```python
from build123d import *

# Parameters (mm, degrees)
F3_DEPTH = 10
F4_R     = 15
F5_DEPTH = 52.4
F6_W     = 100
F6_H     = 6
F7_DEPTH = 18
F8_R     = 10


with BuildPart() as f1:
    # F0 (on Top) → F1 (revolve)
    with BuildSketch(Plane.XY):
        Polygon((-50, 0), (0, 0), (0, 50), (-20, 50), (-20, 30), (-50, 30), align=None)
    revolve(axis=Axis((-25, 0, 0), (1, 0, 0)))

    # F2 (on face) → F3 (cut)
    with BuildSketch(Plane.YZ):
        with BuildLine():
            Line((49.638695, 6), (-49.638695, 6))
            ThreePointArc((-49.638695, 6), (-49.909592, 3.005434), (-50, 0))
            ThreePointArc((-50, 0), (-49.909592, -3.005434), (-49.638695, -6))
            Line((-49.638695, -6), (49.638695, -6))
            ThreePointArc((49.638695, -6), (49.909592, -3.005434), (50, 0))
            ThreePointArc((50, 0), (49.909592, 3.005434), (49.638695, 6))
        make_face()
    extrude(amount=-F3_DEPTH, mode=Mode.SUBTRACT)

    # F4 (on face) → F5 (cut)
    with BuildSketch(Plane(origin=(-50, 0, 0), x_dir=(0, -1, 0), z_dir=(-1, 0, 0))):
        Circle(F4_R)
    extrude(amount=-F5_DEPTH, mode=Mode.SUBTRACT)

    # F6 (on Front) → F7 (cut)
    with BuildSketch(Plane.XZ):
        Rectangle(F6_W, F6_H)
    extrude(amount=-F7_DEPTH, mode=Mode.SUBTRACT)

    # F8
    f8_edges = [f1.edges().sort_by_distance(p)[0] for p in [
        (-20, -30, 0),
    ]]
    fillet(f8_edges, radius=F8_R)


solid = f1.part
```
The listing builds one solid part. Answer for the finished solid, in the listing's coordinates (mm). A direction names the side the tool comes from. Coordinates: 2 decimals unless noted, no trailing zeros. Loops run counter-clockwise (first coordinate to the right, second up) from the corner with the lowest first, then second, coordinate; pieces in that order, holes last. Notation, with made-up numbers: M 79,50 L 91,50 A32 ccw 91,84 Z; hole C -38.75,19 d10. An arc over 180 degrees is marked long. Answer as CSV lines item,"result". Start each with the question number.
(1) The mould has two halves that part along Y. Classify faces 1 (the cylindrical face through (-40.14, -29.97, 1.32)), 2 (the cylindrical face through (-25.35, -14.987, -0.617)), 3 (the flat face through (-5, 32, 6)): pulls with the +Y half, pulls with the -Y half, needs draft (parallel to the pull), parting line crosses it, or undercut.
(2) Given pin 1 (1.5 mm diameter, centred on y = 38.5, z = -23, fed in from -X); pin 2 (12 mm diameter, centred on x = -20, z = 10, fed in from +Y); pin 3 (3 mm diameter, centred on x = -3, y = 25.5, fed in from +Z), each flat-ended and moving along its own axis, determine where each tip first touches the part or whether it passes through.
(3) The part is cut by section C-C (z = 0). Give the vertices of the cut face in (x, y), and give its area (3 significant figures).
(4) The part is cut by section D-D (z = 41.5). Give the vertices of the cut face in (x, y).
(5) Find the intervals of material crossed by L1, parallel to Z at x = -14, y = 0; L2, parallel to Y at x = -13, z = 0; L3, parallel to Z at x = -38, y = 0, in increasing order. Write a range as [from, to].
(6) For faces 4 (the flat face through (-50, 6, 14)), 5 (the flat face through (0, 1, 23)), 6 (the flat face through (-20, -22, 34)), 7 (the flat face through (-30, 16, -3)), 8 (the flat face through (-5, 31, -6)), determine the directions among +Z, -Z, +X, -X, +Y, -Y from which every point of the face is accessible in a straight line to the end or side of a thin tool.
(7) The part is cut by section B-B (y = 0). Give the vertices of the cut face in (x, z).
(8) The part is cut by section A-A (x = -6.5). Give the vertices of the cut face in (y, z), and give its area (3 significant figures).
Determined:
1,face 1,"parting line crosses it"
1,face 2,"undercut"
1,face 3,"needs draft"
2,pin 1,"x = -20"
2,pin 2,"y = 49.84"
2,pin 3,"z = 43.86"
3,outline,"M -50,-30 L -30,-30 A10 cw -20,-40 L -20,-50 L -10,-50 L -10,-15 L -50,-15 Z; M -50,18 L -10,18 L -10,50 L -20,50 L -20,40 A10 cw -30,30 L -50,30 Z"
3,area,"1,520 mm2"
4,outline,"M -20,-27.89 L 0,-27.89 L 0,27.89 L -20,27.89 Z"
5,L1,"[-50, -15], [15, 50]"
5,L2,"[-50, -15], [18, 50]"
5,L3,"[-30, -15], [15, 30]"
6,face 4,"+Z, -Z, -X, +Y, -Y"
6,face 5,"+Z, -Z, +X, +Y, -Y"
6,face 6,"-X"
6,face 7,"+X, -X"
6,face 8,"+X, +Y, -Y"
7,outline,"M -50,-30 L -30,-30 A10 cw -20,-40 L -20,-50 L 0,-50 L 0,-15 L -50,-15 Z; M -50,15 L 0,15 L 0,50 L -20,50 L -20,40 A10 cw -30,30 L -50,30 Z"
8,outline,"M -49.64,-6 A50 ccw 49.64,-6 L 13.75,-6 A15 cw -13.75,-6 Z; M -49.64,6 L -13.75,6 A15 cw 13.75,6 L 49.64,6 A50 ccw Z"
8,area,"6,300 mm2"
